Part model, mm, in its own coordinate system. A direction names the side the tool comes from. Round coordinates to 2 decimals unless told otherwise and drop trailing zeros. Order: outer loops, then holes, each group sorted by start corner. A loop starts at its lowest first (then second) coordinate and runs counter-clockwise, first axis right, second up. Notation, with made-up numbers: (-25.75, -27.5) - (2.25, -27.5) arc R11 ccw to (2.25, -12.5) - close; hole circle Ø1 at (42.5, -30). An arc over 180 degrees is marked (long way). Return JSON: item names as keys, results as strings. Group by question number.
Item 1: Probe probe 1 along Y at (x, z) = (24, 13.25); probe 2 along Z at (x, y) = (63.5, 22); probe 3 along Y at (x, z) = (22.5, 13.5). List the from-to ranges inside material, lowest first.
Item 2: Saw through at C-C on x = 60. State how many separate pieces and enclosed holes the cut face has, and give its area (3 significant figures).
Item 3: Drop flat-ended pins along their axis: pin 1 (6 mm diameter, centred on y = 23, z = 10, fed in from +X); pin 2 (1.8 mm diameter, centred on x = 72.5, z = 13.5, fed in from -Y); pin 3 (2 mm diameter, centred on x = 28.5, y = 13, fed in from -Z). Give the stop position or say it passes through.
Item 4: Tool access for faces 1 (the face through (60, 2.296, 15)), 2 (the face through (59.75, 17.3, 11.59)), 3 (the face through (59.48, 26.953, 16.107)): list every direction of +Z, -Z, +X, -X, +Y, -Y with a clear straight run to the whole face (end or side of a thin tool).
Item 5: Saw through at B-B on z = 13.5. List the corners of the cut face in (x, y).
Item 6: Two-plate mould, pull along X, no slides. Class faces 4 (the face through (59.815, 38.294, 7.19)), 5 (the face through (60, 26, 8.628)), 6 (the face through (61, 13, 17.628)): released by +X, released by -X, zero draft, split by the parting line, or undercut.
Item 7: Saw through at A-A on x = 24. List the corners of the cut face in (y, z), and give its area (3 significant figures).
```python
from build123d import *

# Parameters (mm, degrees)
SKETCH1_R               = 4
BOSS_EXTRUDE1_DEPTH     = 20
SKETCH2_R               = 4
CUT_EXTRUDE1_DEPTH      = 10
FILLET2_R               = 10
CUT_EXTRUDE2_DEPTH      = 5
CUT_EXTRUDE2_DEPTH_BACK = 5
SKETCH5_R               = 20
ECHELLE1_SCALE          = 0.6


with BuildPart() as part:
    # Sketch1 → Boss-Extrude1 (new body)
    with BuildSketch(Plane.XY):
        with BuildLine():
            Line((5.660747058, 13.890858244), (45.074020085, 41.488329122))
            ThreePointArc((45.074020085, 41.488329122), (60, 55), (74.925979915, 41.488329122))
            Line((74.925979915, 41.488329122), (114.339252942, 13.890858244))
            ThreePointArc((114.339252942, 13.890858244), (133.684102891, -6.143722656), (105.857864376, -5))
            Line((105.857864376, -5), (14.142135624, -5))
            ThreePointArc((14.142135624, -5), (-13.684102891, -6.143722656), (5.660747058, 13.890858244))
        make_face()
        with Locations((60, 40)):
            Circle(SKETCH1_R, mode=Mode.SUBTRACT)
        with Locations((120, 0)):
            Circle(SKETCH1_R, mode=Mode.SUBTRACT)
        Circle(SKETCH1_R, mode=Mode.SUBTRACT)
    extrude(amount=BOSS_EXTRUDE1_DEPTH)

    # Sketch2 → Cut-Extrude1 (cut)
    with BuildSketch(Plane(origin=(0, 0, 0), x_dir=(-1, 0, 0), z_dir=(0, 0, -1))):
        with BuildLine():
            ThreePointArc((-40.099720592, 38.00528712), (-60, 20), (-79.900279408, 38.00528712))
            Line((-79.900279408, 38.00528712), (-114.339252942, 13.890858244))
            ThreePointArc((-114.339252942, 13.890858244), (-133.684102891, -6.143722656), (-105.857864376, -5))
            Line((-105.857864376, -5), (-14.142135624, -5))
            ThreePointArc((-14.142135624, -5), (13.684102891, -6.143722656), (-5.660747058, 13.890858244))
            Line((-5.660747058, 13.890858244), (-40.099720592, 38.00528712))
        make_face()
        with Locations((-120, 0)):
            Circle(SKETCH2_R, mode=Mode.SUBTRACT)
        Circle(SKETCH2_R, mode=Mode.SUBTRACT)
    extrude(amount=-CUT_EXTRUDE1_DEPTH, mode=Mode.SUBTRACT)

    # Fillet2
    fillet2_edges = [part.edges().sort_by_distance(p)[0] for p in [
        (60, 20, 10),
    ]]
    fillet(fillet2_edges, radius=FILLET2_R - 0.0001)  # a hair under: the kernel refuses the full size

    # Fillet3: read off the stored shape, not the designer's step
    # Fillet3 outline → Fillet3 (revolve, cut)
    with BuildSketch(Plane(origin=(60, 40, 0), x_dir=(1, 0, 0), z_dir=(0, -1, 0))):
        with BuildLine():
            Line((21.33974599, 0), (21.33974599, 5.000000048))
            ThreePointArc((21.33974599, 5.000000048), (17.679491948, 1.339745976), (12.679491924, 0))
            Line((12.679491924, 0), (21.33974599, 0))
        make_face()
    revolve(axis=Axis((60, 40, 0), (0, 0, 1)), mode=Mode.SUBTRACT)

    # Sketch5 → Cut-Extrude2 (cut, two sides: drawn at the far end of the back side and taken through both)
    with BuildSketch(Plane.XY.offset(10).offset(-CUT_EXTRUDE2_DEPTH_BACK)):
        with Locations((60, 40)):
            Circle(SKETCH5_R)
    extrude(amount=CUT_EXTRUDE2_DEPTH + CUT_EXTRUDE2_DEPTH_BACK, mode=Mode.SUBTRACT)


with BuildPart() as part_1:
    # Echelle1: scaled about (60.000000152, 13.239920992, 14.069971935)
    add(part.part.scale(ECHELLE1_SCALE).moved(Location((24.000000061, 5.295968397, 5.627988774))))


solid = part_1.part
```
Filled in:
{
 "1": {"probe 1": "y = -3.7 to 2.9, 7.7 to 14.3", "probe 2": "z = 5.65 to 8.63, 14.63 to 17.63", "probe 3": "y = -3.58 to 3.42, 7.17 to 14.17"},
 "2": {"separate pieces": "3", "enclosed holes": "0", "area": "192 mm^2"},
 "3": {"pin 1": "stops at x = 82.82", "pin 2": "stops at y = 2.3", "pin 3": "stops at z = 11.63"},
 "4": {"face 1": "+Z, -Z, -Y", "face 2": "+Y", "face 3": "+Z, -Z"},
 "5": {"outline": "(27.4, 13.63) arc R9 ccw (long way) to (32.49, 2.3) - (87.51, 2.3) arc R9 ccw (long way) to (92.6, 13.63) - (71.94, 28.1) arc R12 cw to (48.06, 28.1) - close; hole circle Ø4.8 at (24, 5.3); hole circle Ø4.8 at (96, 5.3)"},
 "6": {"face 4": "split by the parting line", "face 5": "undercut", "face 6": "zero draft"},
 "7": {"outline": "(-3.7, 11.63) - (2.9, 11.63) - (2.9, 17.63) - (-3.7, 17.63) - close; (7.7, 11.63) - (14.3, 11.63) - (14.3, 17.63) - (7.7, 17.63) - close", "area": "79.2 mm^2"}
}
